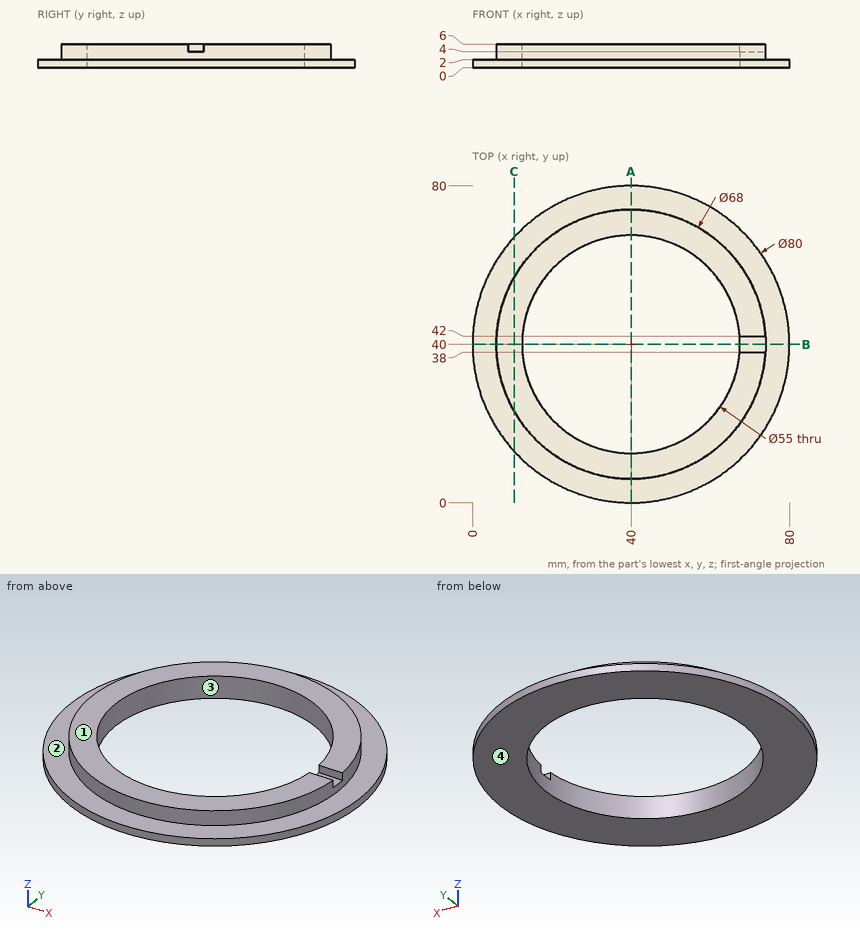
Answer from the drawing. Dimensions are ordinates in mm from the lowest x, y and z of the part. A direction names the side the tool comes from. Coordinates: 2 decimals unless noted, no trailing zeros. Write each loop counter-clockwise with the first axis right and the second up, starting at its lowest first coordinate (ties: lowest second). Pieces come first, ordered by that corner, then holes. Notation, with made-up numbers: (-2, 3) -> (20, 3) arc R20 cw to (20, 38) -> close; hole circle Ø5 at (46, 8.5). An arc over 180 degrees is marked (long way). One line per question, with ' | ' between items.
1. Section B-B (y = 40) is taken. Determine the outline of the cut face in (x, z), and give its area (3 significant figures).
Verdict:
outline: (0, 0) -> (12.5, 0) -> (12.5, 6) -> (6, 6) -> (6, 2) -> (0, 2) -> close; (67.5, 0) -> (80, 0) -> (80, 2) -> (74, 2) -> (74, 4) -> (67.5, 4) -> close | area: 89.0 mm^2
2. Straight lines are drawn through the part: line 1 (X direction, y = 40, z = 2.45); line 2 (Y direction, x = 40, z = 1.7). For each, find the intervals that lie inside material, in ascending order.
Verdict:
line 1: x = 6 to 12.5, 67.5 to 74 | line 2: y = 0 to 12.5, 67.5 to 80
3. For a pull along X with two mould halves and no side action, classify the marked faces 3 and 4 as released by +X, released by -X, zero draft, split by the parting line, or undercut.
Verdict:
face 3: undercut | face 4: zero draft
4. Section C-C (x = 10.5) is taken. Determine the outline of the cut face in (y, z).
Verdict:
outline: (12.99, 0) -> (67.01, 0) -> (67.01, 2) -> (56.9, 2) -> (56.9, 6) -> (23.1, 6) -> (23.1, 2) -> (12.99, 2) -> close
5. Section A-A (x = 40) is taken. Determine the outline of the cut face in (y, z).
Verdict:
outline: (0, 0) -> (12.5, 0) -> (12.5, 6) -> (6, 6) -> (6, 2) -> (0, 2) -> close; (67.5, 0) -> (80, 0) -> (80, 2) -> (74, 2) -> (74, 6) -> (67.5, 6) -> close
6. Given pin 1 Ø3 at (y, z) = (17, 0.5) entering from -X; pin 2 Ø1 at (x, z) = (70, 4.5) entering from +Y; pin 3 Ø2 at (y, z) = (44, 3.5) entering from +X, each flat-ended and moving along its own axis, determine where each tip first touches the part or whether it passes through.
Verdict:
pin 1: stops at x = 6.27 | pin 2: stops at y = 56.9 | pin 3: stops at x = 73.87
7. Which of the six approach directions +Z, -Z, +X, -X, +Y, -Y give full straight-line access (tool end or side, diameter ignored) to the marked faces 1 and 2?
Verdict:
face 1: +Z, +X, -X, +Y, -Y | face 2: +Z
